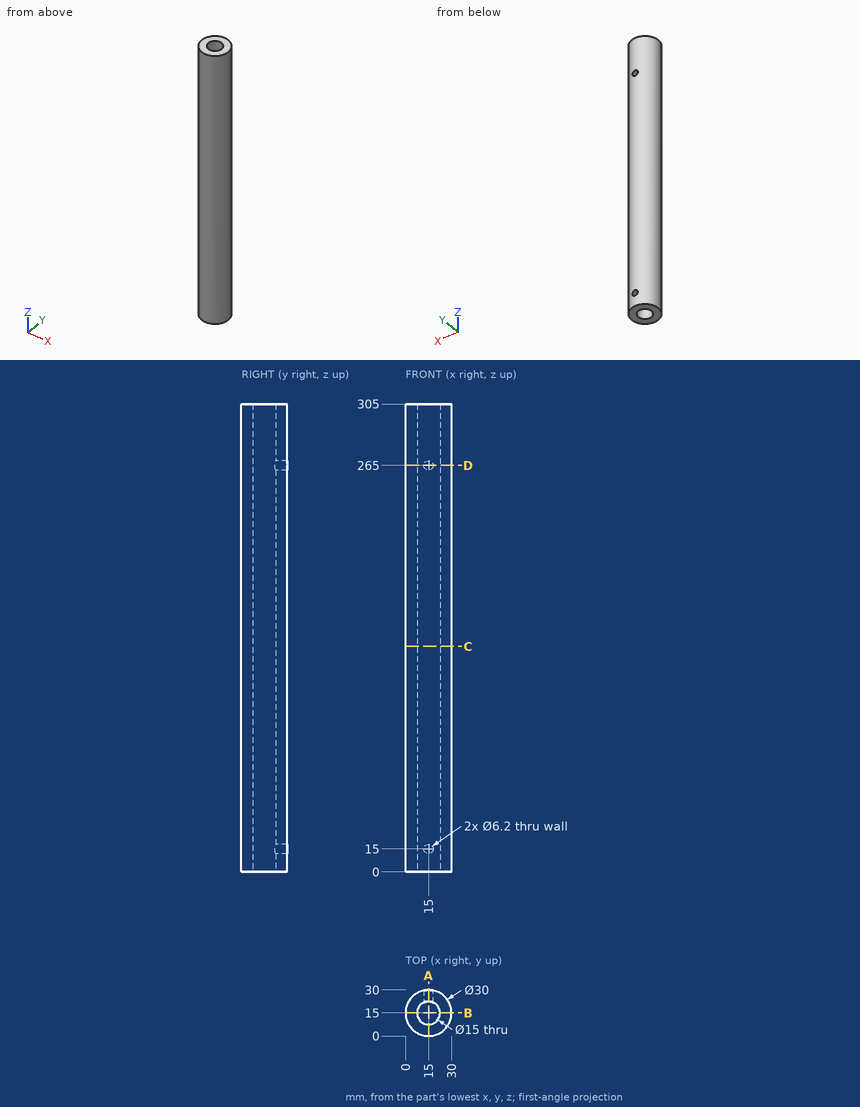
Verification items for this drawing (mm, ordinates from the low corner). Coordinates: 2 decimals unless noted, no trailing zeros. Order: outer loops, then holes, each group sorted by start corner. A loop starts at its lowest first (then second) coordinate and runs counter-clockwise, first axis right, second up.
Q1. Sectioned sample at D-D on z = 265. Record the cut outline in (x, y), and give its area (3 significant figures).
Reply:
outline: (11.9, 21.83) - (11.9, 29.68) arc R15 ccw (long way) to (18.1, 29.68) - (18.1, 21.83) arc R7.5 cw (long way) to start
area: 483 mm2
Q2. Sectioned sample at B-B on y = 15. Record the cut outline in (x, z), and give its area (4 significant figures).
Reply:
outline: (0, 0) - (7.5, 0) - (7.5, 305) - (0, 305) - close; (22.5, 0) - (30, 0) - (30, 305) - (22.5, 305) - close
area: 4,575 mm2
Q3. Sectioned sample at A-A on x = 15. Record the cut outline in (y, z), and give its area (3 significant figures).
Reply:
outline: (0, 0) - (7.5, 0) - (7.5, 305) - (0, 305) - close; (22.5, 0) - (30, 0) - (30, 11.9) - (22.5, 11.9) - close; (22.5, 18.1) - (30, 18.1) - (30, 261.9) - (22.5, 261.9) - close; (22.5, 268.1) - (30, 268.1) - (30, 305) - (22.5, 305) - close
area: 4,480 mm2
Q4. Depth check by flat-ended pin: pin 1 Ø3 at (x, z) = (24, 159) entering from -Y; pin 2 Ø1 at (x, z) = (13.5, 114.5) entering from +Y; pin 3 Ø6 at (x, z) = (19, 105.5) entering from -Y; pin 4 Ø4 at (y, z) = (13.5, 32.5) entering from +X. Enter the tip coordinate at first touch or a pass-through.
Reply:
pin 1: stops at y = 2.01
pin 2: stops at y = 29.97
pin 3: stops at y = 0.03
pin 4: stops at x = 30
Q5. Thickness scan on probe 1 along Z at (x, y) = (15, 26); probe 2 along Y at (x, z) = (15, 154); probe 3 along Y at (x, z) = (9.5, 193). Record the ranges inside material, lowest first.
Reply:
probe 1: z = 0 to 11.9, 18.1 to 261.9, 268.1 to 305
probe 2: y = 0 to 7.5, 22.5 to 30
probe 3: y = 1.04 to 9.9, 20.1 to 28.96
Q6. Sectioned sample at C-C on z = 147. Record the cut outline in (x, y), and give its area (3 significant figures).
Reply:
outline: circle Ø30 at (15, 15); hole circle Ø15 at (15, 15)
area: 530 mm2
